Work out the finished part from the listing and answer in its coordinate system (mm). Round coordinates to 2 decimals unless told otherwise and drop trailing zeros. Order: outer loops, then holes, each group sorted by start corner. A loop starts at its lowest first (then second) coordinate and runs counter-clockwise, first axis right, second up. Notation, with made-up numbers: (17.25, -28.75) -> (62.25, -28.75) arc R27 ccw to (62.25, -10.75) -> close; hole circle Ø10 at (-26, 69). An arc over 180 degrees is marked (long way). Use a Markdown table: item, result. Add a question column.
Item 1: A cutting plane is placed at B-B, the plane y = -114. Determine the outline of the cut face in (x, z), plus the area to 3 significant figures.
Item 2: A cutting plane is placed at C-C, the plane z = -122. Determine the outline of the cut face in (x, y).
Item 3: A cutting plane is placed at A-A, the plane x = 556.5. Determine the outline of the cut face in (y, z), plus the area to 3 significant figures.
Item 4: Find the intervals of material crossed by L1, parallel to Y at x = 155.5, z = -304; L2, parallel to X at y = -137, z = -221.5; L3, parallel to Z at x = -223, y = -107, in increasing order. Write a range as [from, to].
Item 5: Flat-ended cylindrical pins translate along their axes: P1, Ø1.5, axis at x = -39.5, z = -58, coming from the +Y side; P2, Ø8, axis at x = -277.5, z = -104, coming from the -Y side. Find the tip coordinate at first contact, or state that the pin passes through.
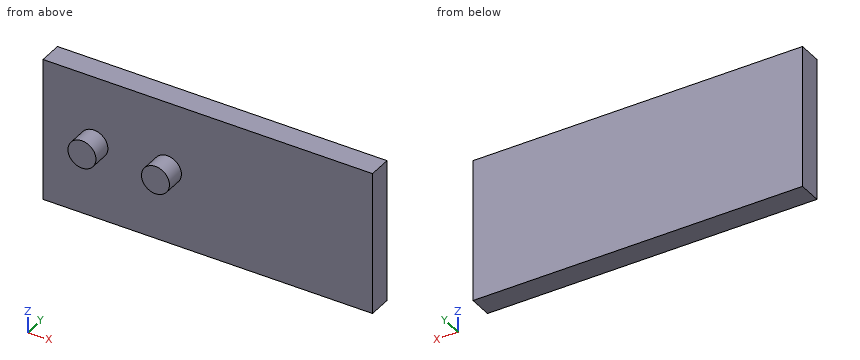
from build123d import *

# Parameters (mm, degrees)
F0_R     = 57.15
F1_DEPTH = 95.2044
F2_R     = 57.15
F3_DEPTH = 173.595728


with BuildPart() as f1:
    # F0 (on Front) → F1 (new body)
    with BuildSketch(Plane.XZ):
        Polygon((662.677174, 75.96576), (-683.522826, 75.96576), (-683.522826, -508.23424), (262.349523, -508.23424), (268.236725, -508.23424), (662.677174, -508.23424), align=None)
        with Locations((-475.626498, -202.36975)):
            Circle(F0_R, mode=Mode.SUBTRACT)
        with BuildLine():
            ThreePointArc((-77.100498, -202.36975), (-134.250498, -259.51975), (-191.400498, -202.36975))
            ThreePointArc((-191.400498, -202.36975), (-134.250498, -145.21975), (-77.100498, -202.36975))
        make_face(mode=Mode.SUBTRACT)
        with Locations((-475.626498, -202.36975)):
            Circle(F0_R)
        with BuildLine():
            ThreePointArc((-77.100498, -202.36975), (-134.250498, -145.21975), (-191.400498, -202.36975))
            ThreePointArc((-191.400498, -202.36975), (-134.250498, -259.51975), (-77.100498, -202.36975))
        make_face()
    extrude(amount=F1_DEPTH)

    # F2 (on Front) + F0 (on Front) → F3 (join)
    with BuildSketch(Plane.XZ):
        with Locations((-175.21213, -203.090936)):
            Circle(F2_R)
    with BuildSketch(Plane.XZ):
        with Locations((-475.626498, -202.36975)):
            Circle(F0_R)
    extrude(amount=F3_DEPTH)


solid = f1.part
Reported:
| question | item | result |
|---|---|---|
| 1 | outline | circle Ø114.3 at (-475.63, -202.37); circle Ø114.3 at (-175.21, -203.09) |
| 1 | area | 20,500 mm² |
| 2 | outline | (-683.52, -95.2) -> (662.68, -95.2) -> (662.68, 0) -> (-683.52, 0) -> close |
| 3 | outline | (-95.2, -508.23) -> (0, -508.23) -> (0, 75.97) -> (-95.2, 75.97) -> close |
| 3 | area | 55,600 mm² |
| 4 | L1 | [-95.2, 0] |
| 4 | L2 | [-529.48, -421.77], [-229.32, -121.11] |
| 4 | L3 | [-234.43, -171.75] |
| 5 | P1 | y = 0 |
| 5 | P2 | y = -95.2 |
